from build123d import *

# Parameters (mm, degrees)
EXTRUDE_1_DEPTH     = 5.5
SKETCH_2_R          = 6.1
CUT_EXTRUDE_1_DEPTH = 2.5
SKETCH_3_R          = 3.5
CUT_EXTRUDE_2_DEPTH = 3
SKETCH_4_R          = 1.7
CUT_EXTRUDE_3_DEPTH = 5.5
SKETCH_5_R          = 5.2
CUT_EXTRUDE_4_DEPTH = 5.5
SKETCH_6_R          = 1.6
SKETCH_6_R_2        = 2.1
CUT_EXTRUDE_5_DEPTH = 5.5
CUT_EXTRUDE_6_DEPTH = 10


with BuildPart() as part:
    # 草图1 → 凸台-拉伸1 (new body)
    with BuildSketch(Plane.XY):
        with BuildLine():
            Line((-48.459116019, -61), (48.459116019, -61))
            ThreePointArc((48.459116019, -61), (53.03620543, -62.438730875), (55.966994877, -66.237436867))
            ThreePointArc((55.966994877, -66.237436867), (69.131727984, -69.131727984), (66.237436867, -55.966994877))
            ThreePointArc((66.237436867, -55.966994877), (62.438730875, -53.03620543), (61, -48.459116019))
            Line((61, -48.459116019), (61, 48.459116019))
            ThreePointArc((61, 48.459116019), (62.438730875, 53.03620543), (66.237436867, 55.966994877))
            ThreePointArc((66.237436867, 55.966994877), (69.131727984, 69.131727984), (55.966994877, 66.237436867))
            ThreePointArc((55.966994877, 66.237436867), (53.03620543, 62.438730875), (48.459116019, 61))
            Line((48.459116019, 61), (25.455844123, 61))
            ThreePointArc((25.455844123, 61), (17.223912036, 64.268717499), (13.476623359, 72.294117647))
            ThreePointArc((13.476623359, 72.294117647), (0, 85), (-13.476623359, 72.294117647))
            ThreePointArc((-13.476623359, 72.294117647), (-17.223912036, 64.268717499), (-25.455844123, 61))
            Line((-25.455844123, 61), (-48.459116019, 61))
            ThreePointArc((-48.459116019, 61), (-53.03620543, 62.438730875), (-55.966994877, 66.237436867))
            ThreePointArc((-55.966994877, 66.237436867), (-69.131727984, 69.131727984), (-66.237436867, 55.966994877))
            ThreePointArc((-66.237436867, 55.966994877), (-62.438730875, 53.03620543), (-61, 48.459116019))
            Line((-61, 48.459116019), (-61, -48.459116019))
            ThreePointArc((-61, -48.459116019), (-62.438730875, -53.03620543), (-66.237436867, -55.966994877))
            ThreePointArc((-66.237436867, -55.966994877), (-69.131727984, -69.131727984), (-55.966994877, -66.237436867))
            ThreePointArc((-55.966994877, -66.237436867), (-53.03620543, -62.438730875), (-48.459116019, -61))
        make_face()
    extrude(amount=-EXTRUDE_1_DEPTH)

    # 草图2 → 切除-拉伸1 (cut)
    with BuildSketch(Plane.XY):
        with Locations((-63.474873734, 63.474873734)):
            Circle(SKETCH_2_R)
        with Locations((63.474873734, 63.474873734)):
            Circle(SKETCH_2_R)
        with Locations((63.474873734, -63.474873734)):
            Circle(SKETCH_2_R)
        with Locations((-63.474873734, -63.474873734)):
            Circle(SKETCH_2_R)
    extrude(amount=-CUT_EXTRUDE_1_DEPTH, mode=Mode.SUBTRACT)

    # 草图3 → 切除-拉伸2 (cut)
    with BuildSketch(Plane.XY.offset(-2.5)):
        with Locations((-63.474873734, 63.474873734)):
            Circle(SKETCH_3_R)
        with Locations((63.474873734, 63.474873734)):
            Circle(SKETCH_3_R)
        with Locations((-63.474873734, -63.474873734)):
            Circle(SKETCH_3_R)
        with Locations((63.474873734, -63.474873734)):
            Circle(SKETCH_3_R)
    extrude(amount=-CUT_EXTRUDE_2_DEPTH, mode=Mode.SUBTRACT)

    # 草图4 → 切除-拉伸3 (cut)
    with BuildSketch(Plane.XY):
        with Locations((8, 71.5)):
            Circle(SKETCH_4_R)
        with Locations((0, 79.5)):
            Circle(SKETCH_4_R)
        with Locations((-8, 71.5)):
            Circle(SKETCH_4_R)
        with Locations((0, 63.5)):
            Circle(SKETCH_4_R)
    extrude(amount=-CUT_EXTRUDE_3_DEPTH, mode=Mode.SUBTRACT)

    # 草图5 → 切除-拉伸4 (cut)
    with BuildSketch(Plane.XY):
        with Locations((0, 71.5)):
            Circle(SKETCH_5_R)
    extrude(amount=-CUT_EXTRUDE_4_DEPTH, mode=Mode.SUBTRACT)

    # 草图6 → 切除-拉伸5 (cut)
    with BuildSketch(Plane.XY):
        with Locations((-40, 40)):
            Circle(SKETCH_6_R)
        with Locations((40, 40)):
            Circle(SKETCH_6_R)
        with Locations((40, -40)):
            Circle(SKETCH_6_R)
        with Locations((-40, -40)):
            Circle(SKETCH_6_R)
        with Locations((-25.5, 25.5)):
            Circle(SKETCH_6_R_2)
        with Locations((25.5, 25.5)):
            Circle(SKETCH_6_R_2)
        with Locations((25.5, -25.5)):
            Circle(SKETCH_6_R_2)
        with Locations((-25.5, -25.5)):
            Circle(SKETCH_6_R_2)
    extrude(amount=-CUT_EXTRUDE_5_DEPTH, mode=Mode.SUBTRACT)

    # 草图8 → 切除-拉伸6 (cut)
    with BuildSketch(Plane.XY):
        with BuildLine():
            Line((4.917472327, 2.796151983), (19.991455189, 17.870134846))
            ThreePointArc((19.991455189, 17.870134846), (21.535572688, 18.451698066), (22.991273845, 17.674878416))
            ThreePointArc((22.991273845, 17.674878416), (29, 0), (22.991273845, -17.674878416))
            ThreePointArc((22.991273845, -17.674878416), (21.535572688, -18.451698066), (19.991455189, -17.870134846))
            Line((19.991455189, -17.870134846), (4.917472327, -2.796151983))
            ThreePointArc((4.917472327, -2.796151983), (4.647578764, -2.30228293), (4.687149257, -1.740871002))
            ThreePointArc((4.687149257, -1.740871002), (5, 0), (4.687149257, 1.740871002))
            ThreePointArc((4.687149257, 1.740871002), (4.647578764, 2.30228293), (4.917472327, 2.796151983))
        make_face()
        with BuildLine():
            Line((2.796151983, 4.917472327), (17.870134846, 19.991455189))
            ThreePointArc((17.870134846, 19.991455189), (18.451698066, 21.535572688), (17.674878416, 22.991273845))
            ThreePointArc((17.674878416, 22.991273845), (0, 29), (-17.674878416, 22.991273845))
            ThreePointArc((-17.674878416, 22.991273845), (-18.451698066, 21.535572688), (-17.870134846, 19.991455189))
            Line((-17.870134846, 19.991455189), (-2.796151983, 4.917472327))
            ThreePointArc((-2.796151983, 4.917472327), (-2.30228293, 4.647578764), (-1.740871002, 4.687149257))
            ThreePointArc((-1.740871002, 4.687149257), (0, 5), (1.740871002, 4.687149257))
            ThreePointArc((1.740871002, 4.687149257), (2.30228293, 4.647578764), (2.796151983, 4.917472327))
        make_face()
        with BuildLine():
            Line((-4.917472327, 2.796151983), (-19.991455189, 17.870134846))
            ThreePointArc((-19.991455189, 17.870134846), (-21.535572688, 18.451698066), (-22.991273845, 17.674878416))
            ThreePointArc((-22.991273845, 17.674878416), (-29, 0), (-22.991273845, -17.674878416))
            ThreePointArc((-22.991273845, -17.674878416), (-21.535572688, -18.451698066), (-19.991455189, -17.870134846))
            Line((-19.991455189, -17.870134846), (-4.917472327, -2.796151983))
            ThreePointArc((-4.917472327, -2.796151983), (-4.647578764, -2.30228293), (-4.687149257, -1.740871002))
            ThreePointArc((-4.687149257, -1.740871002), (-5, 0), (-4.687149257, 1.740871002))
            ThreePointArc((-4.687149257, 1.740871002), (-4.647578764, 2.30228293), (-4.917472327, 2.796151983))
        make_face()
        with BuildLine():
            Line((2.796151983, -4.917472327), (17.870134846, -19.991455189))
            ThreePointArc((17.870134846, -19.991455189), (18.451698066, -21.535572688), (17.674878416, -22.991273845))
            ThreePointArc((17.674878416, -22.991273845), (0, -29), (-17.674878416, -22.991273845))
            ThreePointArc((-17.674878416, -22.991273845), (-18.451698066, -21.535572688), (-17.870134846, -19.991455189))
            Line((-17.870134846, -19.991455189), (-2.796151983, -4.917472327))
            ThreePointArc((-2.796151983, -4.917472327), (-2.30228293, -4.647578764), (-1.740871002, -4.687149257))
            ThreePointArc((-1.740871002, -4.687149257), (0, -5), (1.740871002, -4.687149257))
            ThreePointArc((1.740871002, -4.687149257), (2.30228293, -4.647578764), (2.796151983, -4.917472327))
        make_face()
    extrude(amount=-CUT_EXTRUDE_6_DEPTH, mode=Mode.SUBTRACT)


solid = part.part
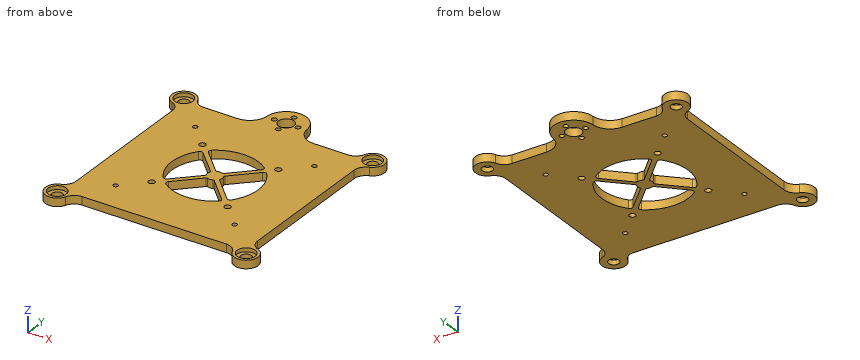
The listing builds one solid part. Answer for the finished solid, in the listing's coordinates (mm). Coordinates: 2 decimals unless noted, no trailing zeros. Loops run counter-clockwise (first coordinate to the right, second up) from the corner with the lowest first, then second, coordinate; pieces in that order, holes last. Notation, with made-up numbers: (-38, 22) -> (21, 22) arc R8 ccw to (21, 32) -> close; hole circle Ø7 at (71, 20). An arc over 180 degrees is marked (long way). Answer in a Markdown table with one row per item. Add a question column.
1. The part is cut by section C-C, the plane y = 25.5. Write down the section's boundary in (x, z).
2. The part is cut by section B-B, the plane y = 79.5. Write down the section's boundary in (x, z).
3. Flat-ended cylindrical pins translate along their axes: P1, Ø1.5, axis at y = -45.5, z = -4.5, coming from the +X side; P2, Ø3, axis at x = 0, y = 79.5, coming from the +Z side; P3, Ø1.5, axis at y = 26, z = -0.5, coming from the -X side; P4, Ø4.5, axis at x = 8, y = 71.5, coming from the +Z side. Find the tip coordinate at first contact, or state that the pin passes through.
4. The part is cut by section D-D, the plane x = -31. Write down the section's boundary in (y, z).
5. Consider line 1 (Y direction, x = 40, z = -5); line 2 (Y direction, x = -63.5, z = -4.4); line 3 (Y direction, x = 10, z = -3). Determine where each line is inside the solid, lowest interval first. Write a range as [from, to].
6. The part is cut by section A-A, the plane x = 0. Write down the section's boundary in (y, z).
Answer below:
| question | item | result |
|---|---|---|
| 1 | outline | (-61, -5.5) -> (-27.6, -5.5) -> (-27.6, 0) -> (-61, 0) -> close; (-23.4, -5.5) -> (-13.81, -5.5) -> (-13.81, 0) -> (-23.4, 0) -> close; (13.81, -5.5) -> (23.4, -5.5) -> (23.4, 0) -> (13.81, 0) -> close; (27.6, -5.5) -> (61, -5.5) -> (61, 0) -> (27.6, 0) -> close |
| 2 | outline | (-10.87, -5.5) -> (-1.7, -5.5) -> (-1.7, 0) -> (-10.87, 0) -> close; (1.7, -5.5) -> (10.87, -5.5) -> (10.87, 0) -> (1.7, 0) -> close |
| 3 | P1 | x = 61 |
| 3 | P2 | through |
| 3 | P3 | x = -61 |
| 3 | P4 | z = 0 |
| 4 | outline | (-61, -5.5) -> (61, -5.5) -> (61, 0) -> (-61, 0) -> close |
| 5 | line 1 | [-61, -41.6], [-38.4, 38.4], [41.6, 61] |
| 5 | line 2 | [-71.47, -66.97], [-59.97, -54.27], [54.27, 59.97], [66.97, 71.47] |
| 5 | line 3 | [-61, -27.22], [-12.12, -7.88], [7.88, 12.12], [27.22, 80.57] |
| 6 | outline | (-61, -5.5) -> (-29, -5.5) -> (-29, 0) -> (-61, 0) -> close; (-5, -5.5) -> (5, -5.5) -> (5, 0) -> (-5, 0) -> close; (29, -5.5) -> (61.8, -5.5) -> (61.8, 0) -> (29, 0) -> close; (65.2, -5.5) -> (66.3, -5.5) -> (66.3, 0) -> (65.2, 0) -> close; (76.7, -5.5) -> (77.8, -5.5) -> (77.8, 0) -> (76.7, 0) -> close; (81.2, -5.5) -> (85, -5.5) -> (85, 0) -> (81.2, 0) -> close |
